Design review of the part shown in the three views and the two pictorial views. Dimensions are in mm from the part's minimum x, y and z. A direction names the side the tool comes from. Round coordinates to 2 decimals unless told otherwise and drop trailing zeros. Order: outer loops, then holes, each group sorted by start corner. A loop starts at its lowest first (then second) coordinate and runs counter-clockwise, first axis right, second up. Notation, with made-up numbers: M -16.75,13.5 L 37.25,13.5 A25 ccw 37.25,44.5 Z; hole C 67.25,-33.5 d11. An arc over 180 degrees is marked long. Write each question's results on one line, items separated by ' | '. Start each with the question number.
Item 1: Wall thickness on line 1 (Y direction, x = 5, z = 3.35); line 2 (Y direction, x = 5, z = 1.6): over which ranges is each line inside the solid? List them lowest first. Write a range as [from, to].
Item 2: Take a section at A-A, the plane x = 5. Write out the cut boundary in (y, z), plus the area to 3 significant figures.
Item 3: Take a section at C-C, the plane y = 2.5. Write out the cut boundary in (x, z).
Item 4: Machinability: for the marked faces 1 and 2, which of the approach directions +Z, -Z, +X, -X, +Y, -Y give a long, thin tool a straight path to every point of the face, cutting with its end or side? Answer none if there is none.
Item 5: Clearance check with flat-ended pins moving along their axes: pin 1 (2 mm diameter, centred on x = 5, y = 5, fed in from -Z); pin 2 (2 mm diameter, centred on x = 4, z = 4.5, fed in from +Y); pin 3 (1 mm diameter, centred on x = 2.5, z = 3.5, fed in from +Y); pin 4 (1 mm diameter, centred on x = 8, z = 3, fed in from +Y). State where each tip first meets the part, or that it passes through.
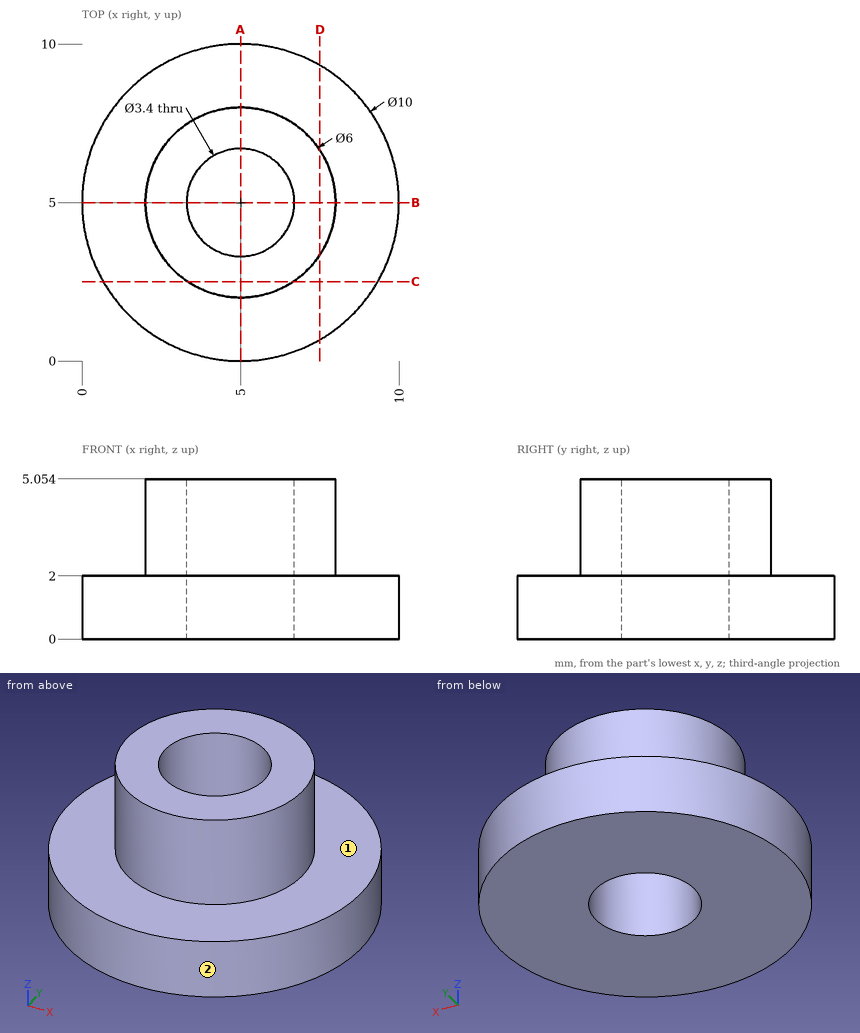
Results list:
1) line 1: [2, 3.3], [6.7, 8] | line 2: [0, 3.3], [6.7, 10]
2) outline: M 0,0 L 3.3,0 L 3.3,5.05 L 2,5.05 L 2,2 L 0,2 Z; M 6.7,0 L 10,0 L 10,2 L 8,2 L 8,5.05 L 6.7,5.05 Z | area: 21.1 mm²
3) outline: M 0.67,0 L 9.33,0 L 9.33,2 L 6.66,2 L 6.66,5.05 L 3.34,5.05 L 3.34,2 L 0.67,2 Z
4) face 1: +Z | face 2: +Z, -Z
5) pin 1: through | pin 2: y = 8 | pin 3: y = 7.24 | pin 4: y = 6.66
